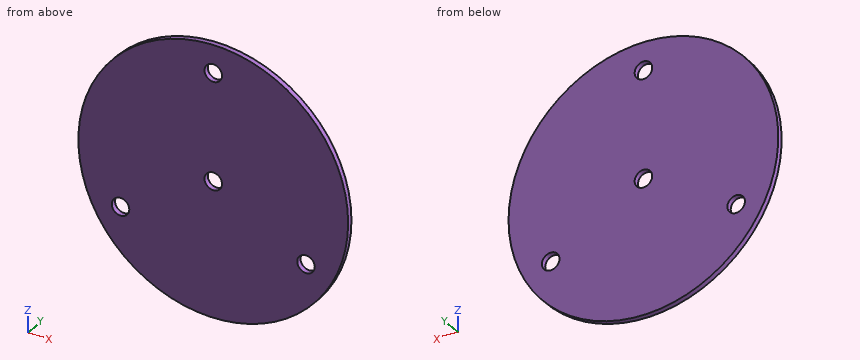
```python
from build123d import *

# Parameters (mm, degrees)
F0_R     = 100
F0_R_2   = 6.5
F1_DEPTH = 4


with BuildPart() as f1:
    # F0 (on Front) → F1 (new body)
    with BuildSketch(Plane.XZ):
        Circle(F0_R)
        with Locations((-68.75, -39.692831)):
            Circle(F0_R_2, mode=Mode.SUBTRACT)
        with Locations((68.75, -39.692831)):
            Circle(F0_R_2, mode=Mode.SUBTRACT)
        Circle(F0_R_2, mode=Mode.SUBTRACT)
        with Locations((0, 79.385662)):
            Circle(F0_R_2, mode=Mode.SUBTRACT)
    extrude(amount=F1_DEPTH)


solid = f1.part
```
Design review of the part built by this model. Coordinates are the model's own, in mm. Give positions to 0.01 mm unless a question says otherwise; leave off trailing zeros. Order: outer loops, then holes, each group sorted by start corner. A loop starts at its lowest first (then second) coordinate and runs counter-clockwise, first axis right, second up. Notation, with made-up numbers: M -20.75,-13.5 L 10.25,-13.5 A24 ccw 10.25,7.5 Z; hole C 63.25,9.25 d2. An arc over 180 degrees is marked long. One line per question, with ' | ' between items. Start each with the question number.
Q1. For L1, parallel to Z at x = 0, y = -3.1; L2, parallel to Z at x = -68.75, y = -2.2; L3, parallel to X at y = -0.85, z = 78, list the stretches that pass through material, from the lowest coordinate up. Write a range as [from, to].
Q2. We need section B-B (z = 0). Write out the cut boundary in (x, y), plus the area to 3 significant figures.
Q3. For pin 1 Ø1 at (y, z) = (-2.5, 14.5) entering from +X, flat-tipped, find the tip position at first contact; note if it passes through.
Q4. We need section D-D (y = -1.8). Write out the cut boundary in (x, z), plus the area to 3 significant figures.
Q5. We need section A-A (x = 0). Write out the cut boundary in (y, z), plus the area to 3 significant figures.
Q6. We need section C-C (x = -69). Write out the cut boundary in (y, z).
Returned:
1) L1: [-100, -6.5], [6.5, 72.89], [85.89, 100] | L2: [-72.62, -46.19], [-33.19, 72.62] | L3: [-62.58, -6.35], [6.35, 62.58]
2) outline: M -100,-4 L -6.5,-4 L -6.5,0 L -100,0 Z; M 6.5,-4 L 100,-4 L 100,0 L 6.5,0 Z | area: 748 mm2
3) pin 1: x = 99.02
4) outline: C 0,0 d200; hole C -68.75,-39.69 d13; hole C 0,0 d13; hole C 0,79.39 d13; hole C 68.75,-39.69 d13 | area: 30,900 mm2
5) outline: M -4,-100 L 0,-100 L 0,-6.5 L -4,-6.5 Z; M -4,6.5 L 0,6.5 L 0,72.89 L -4,72.89 Z; M -4,85.89 L 0,85.89 L 0,100 L -4,100 Z | area: 696 mm2
6) outline: M -4,-72.38 L 0,-72.38 L 0,-46.19 L -4,-46.19 Z; M -4,-33.2 L 0,-33.2 L 0,72.38 L -4,72.38 Z
